from build123d import *

# Parameters (mm, degrees)
SKETCH1_R           = 32
SKETCH1_R_2         = 18
SKETCH1_R_3         = 15
BOSS_EXTRUDE1_DEPTH = 55
SKETCH1_3_R         = 18
SKETCH1_3_R_2       = 15
BOSS_EXTRUDE2_DEPTH = 4
BOSS_EXTRUDE4_START = -55
SKETCH1_6_R         = 18
SKETCH1_6_R_2       = 15
BOSS_EXTRUDE4_DEPTH = 4
SKETCH2_R           = 3
CUT_EXTRUDE1_DEPTH  = 191


with BuildPart() as part:
    # Sketch1 → Boss-Extrude1 (new body)
    with BuildSketch(Plane.XY):
        Circle(SKETCH1_R)
        Circle(SKETCH1_R_2, mode=Mode.SUBTRACT)
        Circle(SKETCH1_R_2)
        Circle(SKETCH1_R_3, mode=Mode.SUBTRACT)
    extrude(amount=-BOSS_EXTRUDE1_DEPTH)

    # Sketch1<3> → Boss-Extrude2 (add)
    with BuildSketch(Plane.XY):
        Circle(SKETCH1_3_R)
        Circle(SKETCH1_3_R_2, mode=Mode.SUBTRACT)
    extrude(amount=BOSS_EXTRUDE2_DEPTH)

    # Sketch1<6> → Boss-Extrude4 (add)
    with BuildSketch(Plane.XY.offset(BOSS_EXTRUDE4_START)):
        Circle(SKETCH1_6_R)
        Circle(SKETCH1_6_R_2, mode=Mode.SUBTRACT)
    extrude(amount=-BOSS_EXTRUDE4_DEPTH)

    # Sketch2 → Cut-Extrude1 (cut)
    with BuildSketch(Plane.XY):
        with Locations((-16.970562748, 16.970562748)):
            Circle(SKETCH2_R)
        with Locations((16.970562748, 16.970562748)):
            Circle(SKETCH2_R)
        with Locations((16.970562748, -16.970562748)):
            Circle(SKETCH2_R)
        with Locations((-16.970562748, -16.970562748)):
            Circle(SKETCH2_R)
    extrude(amount=-CUT_EXTRUDE1_DEPTH, mode=Mode.SUBTRACT)


solid = part.part
CAD build for the part. Positions are in the model's coordinates, mm. A direction names the side the tool comes from. Round coordinates to 2 decimals unless told otherwise and drop trailing zeros. Loops run counter-clockwise (first coordinate to the right, second up) from the corner with the lowest first, then second, coordinate; pieces in that order, holes last.
(1) Drop flat-ended pins along their axis: pin 1 (7 mm diameter, centred on x = 16.97, y = 16.97, fed in from +Z); pin 2 (12 mm diameter, centred on x = -10.5, z = -24.5, fed in from -Y); pin 3 (2 mm diameter, centred on y = -24.5, z = -6, fed in from -X). Give the stop position or say it passes through.
(2) Which spindle directions (+Z, -Z, +X, -X, +Y, -Y) get a long thin tool onto all of the face, cutting with end or side? Do faces 5 (the cylindrical face through (-14.985, 0.66, -27.059)), 6 (the flat face through (14, -14, 0)). Say none if no direction does.
(3) Cut at C-C (z = -17.5). Give the cut face in (x, y), plus the area to 3 significant figures.
(4) Cut at A-A (y = 0). Give the cut face in (x, z).
(5) Cut at D-D (y = 27.5). Give the cut face in (x, z), plus the area to 3 significant figures.
(6) Two-plate mould, pull along Y, no slides. Class faces 1 (the cylindrical face through (-17.62, -19.9, -27.12)), 2 (the cylindrical face through (-2.343, 17.847, -56.972)), 3 (the flat face through (14, -14, -55)), 4 (the cylindrical face through (16.32, -19.9, -27.12)): +Y half, -Y half, draft (parallel to the pull), parting line (faces both ways), or undercut.
(7) Wall check: line 1 along Y through (x, z) = (0, -43); line 2 along X through (y, z) = (16, -43.5). Give the ranges that are in metal, low to high.
Findings below:
1. pin 1: stops at z = 0
1. pin 2: stops at y = -31.68
1. pin 3: stops at x = -21.72
2. face 5: +Z, -Z
2. face 6: +Z
3. outline: circle Ø64 at (0, 0); hole circle Ø6 at (-16.97, -16.97); hole circle Ø6 at (-16.97, 16.97); hole circle Ø30 at (0, 0); hole circle Ø6 at (16.97, -16.97); hole circle Ø6 at (16.97, 16.97)
3. area: 2,400 mm2
4. outline: (-32, -55) - (-18, -55) - (-18, -59) - (-15, -59) - (-15, 4) - (-18, 4) - (-18, 0) - (-32, 0) - close; (15, -59) - (18, -59) - (18, -55) - (32, -55) - (32, 0) - (18, 0) - (18, 4) - (15, 4) - close
5. outline: (-16.36, -55) - (16.36, -55) - (16.36, 0) - (-16.36, 0) - close
5. area: 1,800 mm2
6. face 1: undercut
6. face 2: parting line
6. face 3: draft
6. face 4: undercut
7. line 1: y = -32 to -15, 15 to 32
7. line 2: x = -27.71 to -19.81, -14.13 to 14.13, 19.81 to 27.71
